Print and shaded views of the part. All mm, measured from the part's lowest x, y and z. Round coordinates to 2 decimals unless told otherwise and drop trailing zeros. Order: outer loops, then holes, each group sorted by start corner. A loop starts at its lowest first (then second) coordinate and runs counter-clockwise, first axis right, second up.
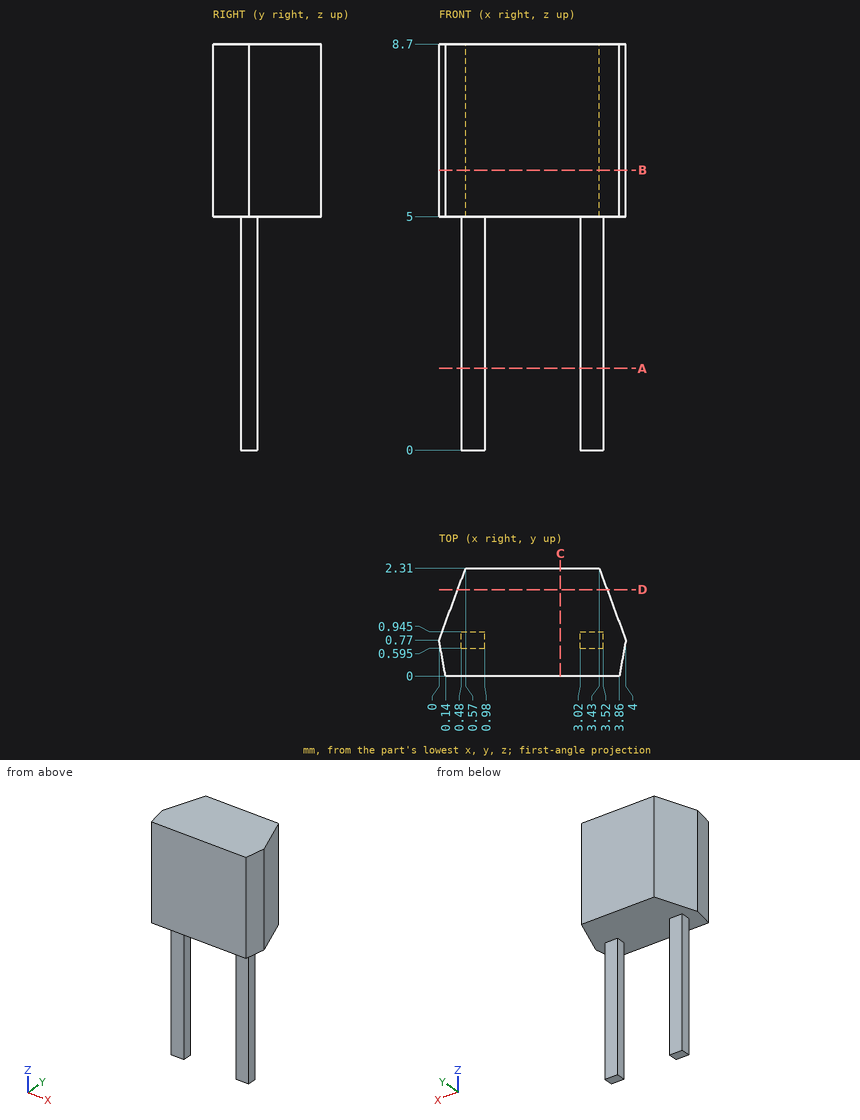
1. Cut at B-B, the plane z = 6. Write the cut outline in (x, y), and give its area (3 significant figures).
2. Cut at D-D, the plane y = 1.85. Write the cut outline in (x, z), and give its area (3 significant figures).
3. Cut at A-A, the plane z = 1.75. Write the cut outline in (x, y) (3 decimals), and give its area (3 significant figures).
4. Drill centre lines: line 1 (X direction, y = 0.75, z = 4.25); line 2 (Z direction, x = 0.45, y = 0.3); line 3 (X direction, y = 0.9, z = 6). Where is each one in solid material? Low to high.
5. Cut at C-C, the plane x = 2.6. Write the cut outline in (y, z), and give its area (3 significant figures).
6. Pin check, flat tips, straight feed: P1, Ø0.6, axis at x = 0.5, z = 2.5, coming from the +Y side (3 decimals); P2, Ø1, axis at y = 2, z = 6, coming from the -X side; P3, Ø0.6, axis at x = 0.5, z = 3.5, coming from the -Y side (3 decimals). Stop position of each tip, or through.
Outcome:
1. outline: (0, 0.77) - (0.14, 0) - (3.86, 0) - (4, 0.77) - (3.43, 2.31) - (0.57, 2.31) - close
1. area: 8.25 mm2
2. outline: (0.4, 5) - (3.6, 5) - (3.6, 8.7) - (0.4, 8.7) - close
2. area: 11.8 mm2
3. outline: (0.48, 0.595) - (0.98, 0.595) - (0.98, 0.945) - (0.48, 0.945) - close; (3.02, 0.595) - (3.52, 0.595) - (3.52, 0.945) - (3.02, 0.945) - close
3. area: 0.350 mm2
4. line 1: x = 0.48 to 0.98, 3.02 to 3.52
4. line 2: z = 5 to 8.7
4. line 3: x = 0.05 to 3.95
5. outline: (0, 5) - (2.31, 5) - (2.31, 8.7) - (0, 8.7) - close
5. area: 8.55 mm2
6. P1: stops at y = 0.945
6. P2: stops at x = 0.27
6. P3: stops at y = 0.595
